```python
from build123d import *

# Parameters (mm, degrees)
F0_R     = 35
F1_DEPTH = 10
F2_R     = 25
F3_DEPTH = 25
F4_W     = 20
F4_H     = 80
F5_DEPTH = 25
F7_R     = 32.5
F7_R_2   = 22.5
F8_DEPTH = 1


with BuildPart() as f1:
    # F0 (on Top) → F1 (new body)
    with BuildSketch(Plane.XY):
        Circle(F0_R)
    extrude(amount=F1_DEPTH)

    # F2 (on Top) → F3 (join)
    with BuildSketch(Plane.XY):
        Circle(F2_R)
    extrude(amount=-F3_DEPTH)

    # F4 (on Top) → F5 (cut)
    with BuildSketch(Plane.XY):
        Rectangle(F4_W, F4_H)
    extrude(amount=-F5_DEPTH, mode=Mode.SUBTRACT)

    # F7 (on offset) → F8 (cut)
    with BuildSketch(Plane.XY.offset(10)):
        Circle(F7_R)
        Circle(F7_R_2, mode=Mode.SUBTRACT)
    extrude(amount=-F8_DEPTH, mode=Mode.SUBTRACT)


solid = f1.part
```
Work out the finished part from the listing and answer in its coordinate system (mm). A direction names the side the tool comes from. Round coordinates to 2 decimals unless told otherwise and drop trailing zeros. Loops run counter-clockwise (first coordinate to the right, second up) from the corner with the lowest first, then second, coordinate; pieces in that order, holes last. Notation, with made-up numbers: M 2,-17.75 L 54,-17.75 A14 ccw 54,3.25 Z; hole C 48.5,57 d8. An arc over 180 degrees is marked long. Use CSV: the item, a comma, the result in double quotes.
Q1. Consider L1, parallel to Y at x = 0, z = 9.6; L2, parallel to Z at x = 7.5, y = -7; L3, parallel to Z at x = -17.5, y = -27. Determine where each line is inside the solid, lowest interval first.
Determined:
L1,"-35 to -32.5, -22.5 to 22.5, 32.5 to 35"
L2,"0 to 10"
L3,"0 to 9"
Q2. Section D-D, the plane z = 2.5 is taken. Determine the outline of the cut face in (x, y).
Determined:
outline,"C 0,0 d70"
Q3. Section A-A, the plane x = 0 is taken. Determine the outline of the cut face in (y, z).
Determined:
outline,"M -35,0 L 35,0 L 35,10 L 32.5,10 L 32.5,9 L 22.5,9 L 22.5,10 L -22.5,10 L -22.5,9 L -32.5,9 L -32.5,10 L -35,10 Z"
Q4. Section C-C, the plane z = -22 is taken. Determine the outline of the cut face in (x, y), then the cut area to 3 significant figures.
Determined:
outline,"M -10,-22.91 L -10,22.91 A25 ccw Z; M 10,-22.91 A25 ccw 10,22.91 Z"
area,"991 mm2"
Q5. Each of these flat-tipped pins is pushed along its axis until it touches: pin 1 (12.5 mm diameter, centred on y = 2, z = -6.5, fed in from +X); pin 2 (2 mm diameter, centred on y = -21.5, z = -12, fed in from -X); pin 3 (1.5 mm diameter, centred on x = -23.5, z = 5.5, fed in from -Y). Where does it stop, or does it pass through?
Determined:
pin 1,"x = 25"
pin 2,"x = -14.31"
pin 3,"y = -26.6"
Q6. The mould has two halves that part along Y. Classify faces 6 (the cylindrical face through (25, 0, -12)), 7 (the flat face through (7, 22, 9)), 8 (the flat face through (10, 0, -12)): pulls with the +Y half, pulls with the -Y half, needs draft (parallel to the pull), parting line crosses it, or undercut.
Determined:
face 6,"parting line crosses it"
face 7,"undercut"
face 8,"needs draft"
Q7. Section B-B, the plane y = 0 is taken. Determine the outline of the cut face in (x, z).
Determined:
outline,"M -35,0 L -25,0 L -25,-25 L -10,-25 L -10,0 L 10,0 L 10,-25 L 25,-25 L 25,0 L 35,0 L 35,10 L 32.5,10 L 32.5,9 L 22.5,9 L 22.5,10 L -22.5,10 L -22.5,9 L -32.5,9 L -32.5,10 L -35,10 Z"
Q8. A tool of negligible diameter and unlimited length cuts with its end or side. For faces 1 (the flat face through (-10, 0, -12)), 2 (the cylindrical face through (-25, 0, -12)), 3 (the cylindrical face through (31, 9.76, 9.51)), 4 (the cylindrical face through (-28, -21, 5)), 5 (the flat face through (-16, 0, -25)), from which of +Z, -Z, +X, -X, +Y, -Y can it reach the whole face along a straight path? Write none if from no direction.
Determined:
face 1,"-Z, +Y, -Y"
face 2,"-Z, -X"
face 3,"+Z"
face 4,"+Z, -Z"
face 5,"-Z, +X, -X, +Y, -Y"
